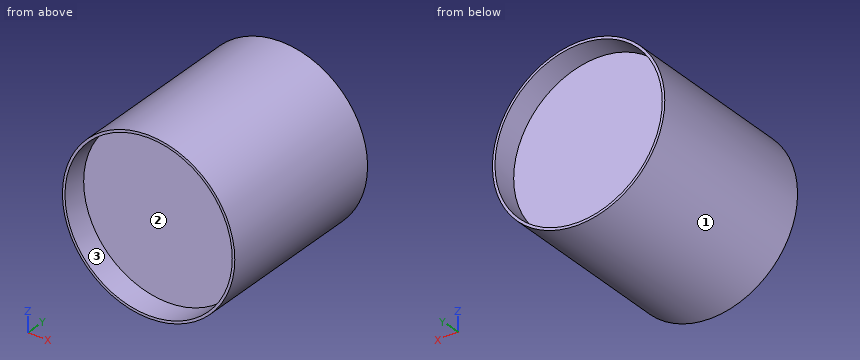
```python
from build123d import *

# Parameters (mm, degrees)
SKETCH1_R           = 34
SKETCH1_R_2         = 33
BOSS_EXTRUDE1_DEPTH = 71
SKETCH2_W           = 33
SKETCH2_H           = 51


with BuildPart() as part:
    # Sketch1 → Boss-Extrude1 (new body)
    with BuildSketch(Plane(origin=(0, 0, 0), x_dir=(1, 0, 0), z_dir=(0, 1, 0))):
        with Locations(Location((0, 0, 0), (0, 0, 270))):
            Circle(SKETCH1_R)
        with Locations(Location((0, 0, 0), (0, 0, 270))):
            Circle(SKETCH1_R_2, mode=Mode.SUBTRACT)
    extrude(amount=BOSS_EXTRUDE1_DEPTH)

    # Sketch2 → Revolve1 (revolve)
    with BuildSketch(Plane.XY, mode=Mode.PRIVATE) as revolve1_sk:
        with Locations((-16.5, 35.5)):
            Rectangle(SKETCH2_W, SKETCH2_H)
    revolve(revolve1_sk.sketch.rotate(Axis((0, 61, 0), (0, -1, 0)), 90), axis=Axis((0, 61, 0), (0, -1, 0)))


solid = part.part
```
Here's how the part is built. I have some questions about the finished solid (model axes, mm). Face numbers are marked on the shaded views. Coordinates: 2 decimals unless noted, no trailing zeros. Write each loop counter-clockwise with the first axis right and the second up, starting at its lowest first coordinate (ties: lowest second). Pieces come first, ordered by that corner, then holes. Notation, with made-up numbers: (-18.75, 61) -> (1.25, 61) arc R27 cw to (1.25, 94) -> close; hole circle Ø4 at (27, 19.25). An arc over 180 degrees is marked (long way). Use a Markdown table: item, result. Add a question column.
(1) If we section it at B-B, the plane z = 0: Write out the boundary of the cut face in (x, y).
(2) Please list where these lines run through material, in increasing order: line 1 (X direction, y = 67.25, z = 0); line 2 (Y direction, x = 19, z = -10.5); line 3 (Z direction, x = 25, y = 22).
(3) If we section it at C-C, the plane y = 40: Write out the boundary of the cut face in (x, z).
(4) We'd pull the mould along Z, two halves only. Please class the marked faces 1, 2 and 3: +Z half, -Z half, draft (parallel to the pull), parting line (faces both ways), or undercut.
(5) If we section it at A-A, the plane x = 0: Write out the boundary of the cut face in (y, z), and give its area (3 significant figures).
(6) I'm going to push flat-ended pins straight in: P1, Ø10, axis at y = 21.5, z = -2, coming from the +X side; P2, Ø20, axis at x = 15, z = 12, coming from the -Y side; P3, Ø3, axis at x = -15.5, z = 19.5, coming from the +Y side. Where does each tip first touch, or does it pass through?
Outcome:
| question | item | result |
|---|---|---|
| 1 | outline | (-34, 0) -> (-33, 0) -> (-33, 10) -> (33, 10) -> (33, 0) -> (34, 0) -> (34, 71) -> (33, 71) -> (33, 61) -> (-33, 61) -> (-33, 71) -> (-34, 71) -> close |
| 2 | line 1 | x = -34 to -33, 33 to 34 |
| 2 | line 2 | y = 10 to 61 |
| 2 | line 3 | z = -23.04 to 23.04 |
| 3 | outline | circle Ø68 at (0, 0) |
| 4 | face 1 | parting line |
| 4 | face 2 | undercut |
| 4 | face 3 | undercut |
| 5 | outline | (0, -34) -> (71, -34) -> (71, -33) -> (61, -33) -> (61, 33) -> (71, 33) -> (71, 34) -> (0, 34) -> (0, 33) -> (10, 33) -> (10, -33) -> (0, -33) -> close |
| 5 | area | 3,510 mm^2 |
| 6 | P1 | stops at x = 34 |
| 6 | P2 | stops at y = 10 |
| 6 | P3 | stops at y = 61 |
